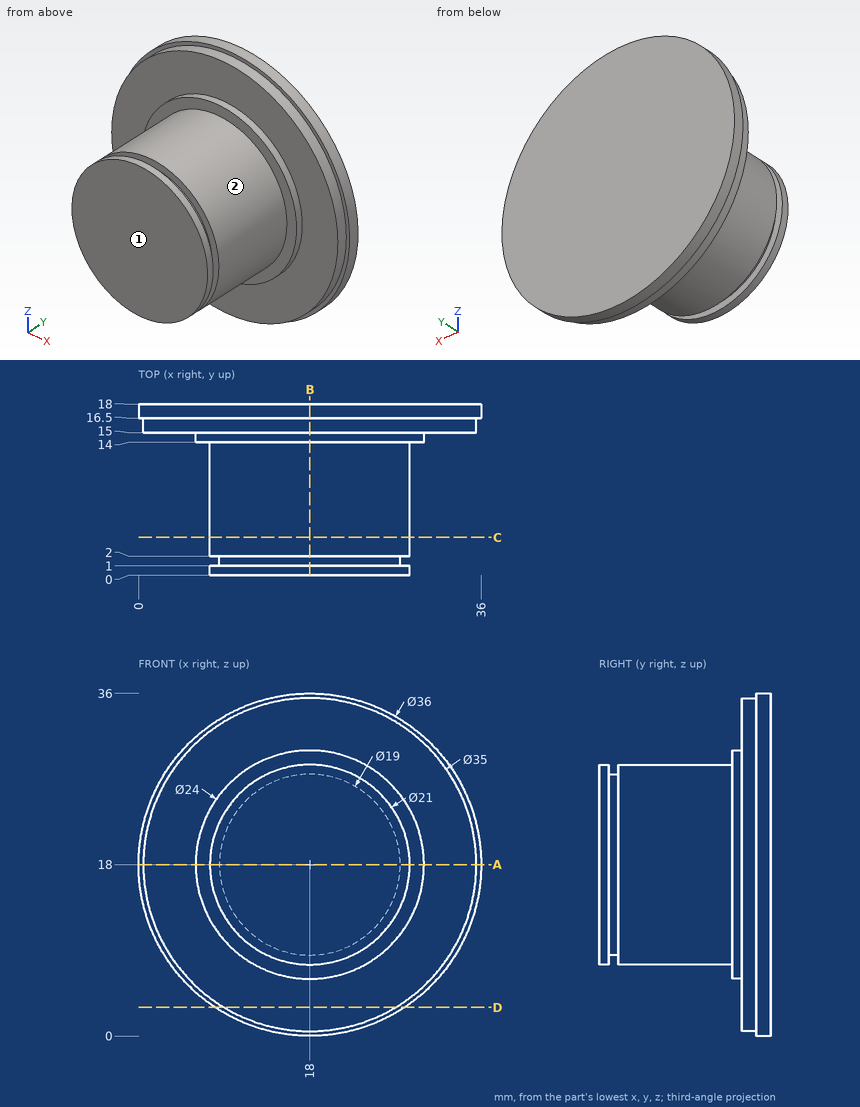
Answer from the drawing. Dimensions are ordinates in mm from the lowest x, y and z of the part. A direction names the side the tool comes from. Give positions to 0.01 mm unless a question says otherwise; leave off trailing zeros. Order: outer loops, then holes, each group sorted by start corner. A loop starts at its lowest first (then second) coordinate and runs counter-clockwise, first axis right, second up. Notation, with made-up numbers: (54.25, -15.5) -> (102.25, -15.5) arc R19 cw to (102.25, 11.5) -> close; hole circle Ø6 at (81.5, 67). An arc over 180 degrees is marked (long way). Answer as a JSON object with one key per item and string values. Group by question number.
1. Consider line 1 along Y through (x, z) = (5.5, 9.5); line 2 along Y through (x, z) = (29, 17.5); line 3 along Z through (x, y) = (11, 4.5). Determine where each line is inside the solid, lowest interval first. Write a range as [from, to].
2. Section C-C on y = 4 is taken. Determine the outline of the cut face in (x, z).
3. Section A-A on z = 18 is taken. Determine the outline of the cut face in (x, y), plus the area to 4 significant figures.
4. Section D-D on z = 3 is taken. Determine the outline of the cut face in (x, y).
5. Flat-ended cylindrical pins translate along their axes: pin 1 Ø10 at (x, y) = (14, 4.5) entering from -Z; pin 2 Ø10.5 at (x, z) = (15.5, 15.5) entering from -Y; pin 3 Ø10 at (y, z) = (13, 29.5) entering from -X; pin 4 Ø1 at (y, z) = (3.5, 23) entering from -X. Find the tip coordinate at first contact, or state that the pin passes through.
6. A tool of negligible diameter and unlimited length cuts with its end or side. For the marked faces 1 and 2, from which of +Z, -Z, +X, -X, +Y, -Y can it reach the whole face along a straight path? Write none if from no direction.
7. Section B-B on x = 18 is taken. Determine the outline of the cut face in (y, z), plus the area to 4 significant figures.
Result sheet:
{
 "1": {"line 1": "y = [15, 18]", "line 2": "y = [14, 18]", "line 3": "z = [10.17, 25.83]"},
 "2": {"outline": "circle Ø21 at (18, 18)"},
 "3": {"outline": "(0, 16.5) -> (0.5, 16.5) -> (0.5, 15) -> (6, 15) -> (6, 14) -> (7.5, 14) -> (7.5, 2) -> (8.5, 2) -> (8.5, 1) -> (7.5, 1) -> (7.5, 0) -> (28.5, 0) -> (28.5, 1) -> (27.5, 1) -> (27.5, 2) -> (28.5, 2) -> (28.5, 14) -> (30, 14) -> (30, 15) -> (35.5, 15) -> (35.5, 16.5) -> (36, 16.5) -> (36, 18) -> (0, 18) -> close", "area": "422.5 mm^2"},
 "4": {"outline": "(8.05, 16.5) -> (8.99, 16.5) -> (8.99, 15) -> (27.01, 15) -> (27.01, 16.5) -> (27.95, 16.5) -> (27.95, 18) -> (8.05, 18) -> close"},
 "5": {"pin 1": "stops at z = 7.5", "pin 2": "stops at y = 0", "pin 3": "stops at x = 1.84", "pin 4": "stops at x = 8.51"},
 "6": {"face 1": "+Z, -Z, +X, -X, -Y", "face 2": "-Y"},
 "7": {"outline": "(0, 7.5) -> (1, 7.5) -> (1, 8.5) -> (2, 8.5) -> (2, 7.5) -> (14, 7.5) -> (14, 6) -> (15, 6) -> (15, 0.5) -> (16.5, 0.5) -> (16.5, 0) -> (18, 0) -> (18, 36) -> (16.5, 36) -> (16.5, 35.5) -> (15, 35.5) -> (15, 30) -> (14, 30) -> (14, 28.5) -> (2, 28.5) -> (2, 27.5) -> (1, 27.5) -> (1, 28.5) -> (0, 28.5) -> close", "area": "422.5 mm^2"}
}
